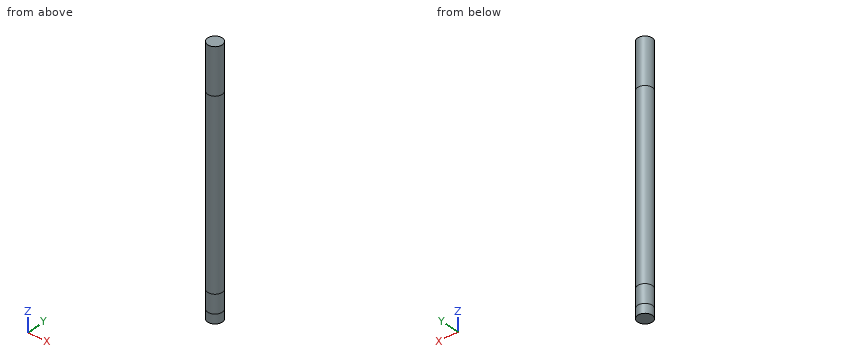
Autodesk Inventor part; units mm, degrees
ref_plane "YZ Plane" through (0, 0, 0) normal (1, 0, 0) x (0, 1, 0)
ref_plane "XZ Plane" through (0, 0, 0) normal (0, 1, 0) x (-1, 0, 0)
ref_plane "XY Plane" through (0, 0, 0) normal (0, 0, 1) x (1, 0, 0)
sketch "スケッチ1" plane through (0, 0, 0) normal (0, 0, 1) x (1, 0, 0)
  circle A0 centre (0, 0) radius 4
  dimension "d0" = 8
extrude "押し出し1" add sketch "スケッチ1" along normal blind 100
sketch "スケッチ2" plane through (0, 0, 0) normal (0, 0, -1) x (-1, 0, 0)
  circle A0 centre (0, 0) radius 4
extrude "押し出し2" add sketch "スケッチ2" along normal blind 10
sketch "スケッチ3" plane through (0, 0, 100) normal (0, 0, 1) x (1, 0, 0)
  circle A0 centre (0, 0) radius 4
  circle A1 centre (0, 0) radius 4
  dimension "d5" = 8
extrude "押し出し3" add sketch "スケッチ3" along normal blind 25
sketch "スケッチ4" plane through (0, 0, -10) normal (0, 0, -1) x (-1, 0, 0)
  circle A0 centre (0, 0) radius 4
extrude "押し出し4" add sketch "スケッチ4" along normal blind 5
properties part number "8mm軸_2"
The model under review builds one solid part; all positions refer to its coordinate system, in mm. Round coordinates to 2 decimals unless told otherwise and drop trailing zeros. Order: outer loops, then holes, each group sorted by start corner. A loop starts at its lowest first (then second) coordinate and runs counter-clockwise, first axis right, second up. Notation, with made-up numbers: (60, -39) - (85, -39) arc R11 ccw to (85, -21) - close; hole circle Ø6 at (12.25, 69). An arc over 180 degrees is marked (long way). Answer in a Markdown table with one row per item.
(1) Take a section at C-C on y = 1.75. Write out the cut boundary in (x, z), plus the area to 3 significant figures.
Result set:
| item | result |
|---|---|
| outline | (-3.6, -15) - (3.6, -15) - (3.6, 125) - (-3.6, 125) - close |
| area | 1,010 mm2 |
(2) Clearance check with flat-ended pins moving along their axes: P1, Ø2, axis at y = -1.5, z = 99.5, coming from the -X side; P2, Ø4, axis at x = -3, z = 106, coming from the +Y side. State where each tip first meets the part, or that it passes through.
Result set:
| item | result |
|---|---|
| P1 | stops at x = -3.97 |
| P2 | stops at y = 3.87 |
(3) For line 1 (Y direction, x = 2.5, z = 104); line 2 (Y direction, x = -3, z = 69.5); line 3 (X direction, y = 0.25, z = 60), list the stretches that pass through material, from the lowest coordinate up. Write a range as from..to.
Result set:
| item | result |
|---|---|
| line 1 | y = -3.12..3.12 |
| line 2 | y = -2.65..2.65 |
| line 3 | x = -3.99..3.99 |
(4) Take a section at A-A on z = 92. Write out the cut boundary in (x, y).
Result set:
| item | result |
|---|---|
| outline | circle Ø8 at (0, 0) |
(5) Take a section at B-B on x = -1.25. Write out the cut boundary in (y, z), plus the area to 3 significant figures.
Result set:
| item | result |
|---|---|
| outline | (-3.8, -15) - (3.8, -15) - (3.8, 125) - (-3.8, 125) - close |
| area | 1,060 mm2 |
